Can you work these out from the model? Positions are in its coordinate system, mm. Give positions to 0.01 mm unless a question says otherwise; leave off trailing zeros. Order: outer loops, then holes, each group sorted by start corner. A loop starts at its lowest first (then second) coordinate and runs counter-clockwise, first axis right, second up. Notation, with made-up numbers: (63.25, 75.25) - (83.25, 75.25) arc R15 cw to (83.25, 104.25) - close; hole circle Ø4 at (39.5, 79.25). An arc over 180 degrees is marked (long way). Use one line per item in the form item = value. Start each with the question number.
1) Suppose I cut it at C-C, the plane y = 1405. Write out the boundary of the cut face in (x, z), and give its area (3 significant figures).
2) For pin 1 (10 mm diameter, centred on y = 260, z = 84, fed in from -X); pin 2 (2 mm diameter, centred on x = 2.5, y = 1288, fed in from +Z); pin 3 (1 mm diameter, centred on y = 208.5, z = -30, fed in from -X), each with a flat end and sliding along its axis, tell me the tip position at first contact or that it passes through.
3) Please list where these lines run through material, in increasing order: probe 1 along X at (y, z) = (1181, -28.5); probe 2 along X at (y, z) = (198, -17.5); probe 3 along Z at (x, y) = (-104, 310).
4) Suppose I cut it at B-B, the plane x = 101. Write out the boundary of the cut face in (y, z), and give its area (3 significant figures).
5) Suppose I cut it at D-D, the plane x = 0. Write out the boundary of the cut face in (y, z).
6) Suppose I cut it at A-A, the plane z = -27. Write out the boundary of the cut face in (x, y).
```python
from build123d import *

# Parameters (mm, degrees)
BOSS_EXTRUDE1_DEPTH = 1510


with BuildPart() as part:
    # Sketch2 → Boss-Extrude1 (new body)
    with BuildSketch(Plane(origin=(0, 0, 0), x_dir=(1, 0, 0), z_dir=(0, 1, 0))):
        with BuildLine():
            ThreePointArc((70.554092404, 97.067605539), (106.926355704, 54.467921346), (120, 0))
            Line((120, 0), (125, 0))
            ThreePointArc((125, 0), (111.381620526, 56.737418069), (73.493846254, 101.112089103))
            Line((73.493846254, 101.112089103), (70.554092404, 97.067605539))
        make_face()
        with BuildLine():
            Line((-125, 0), (-120, 0))
            ThreePointArc((-120, 0), (-114.122987747, 37.093714665), (-97.067605539, 70.554092404))
            Line((-97.067605539, 70.554092404), (-101.112089103, 73.493846254))
            ThreePointArc((-101.112089103, 73.493846254), (-118.878112237, 38.63928611), (-125, 0))
        make_face()
        with BuildLine():
            Line((125, 0), (120, 0))
            ThreePointArc((120, 0), (0, -120), (-120, 0))
            Line((-120, 0), (-125, 0))
            ThreePointArc((-125, 0), (0, -125), (125, 0))
        make_face()
    extrude(amount=BOSS_EXTRUDE1_DEPTH)


solid = part.part
```
Result sheet:
q1.outline = (-101.11, -73.49) - (-97.07, -70.55) arc R120 cw (long way) to (70.55, -97.07) - (73.49, -101.11) arc R125 ccw (long way) to start
q1.area = 2,890 mm²
q2.pin_1 = -96.87
q2.pin_2 = 124.99
q2.pin_3 = -121.47
q3.probe_1 = -121.71 to -116.57, 116.57 to 121.71
q3.probe_2 = -123.77 to -118.72, 118.72 to 123.77
q3.probe_3 = -69.35 to -59.87, 59.87 to 69.35
q4.outline = (0, -73.65) - (1510, -73.65) - (1510, -64.8) - (0, -64.8) - close; (0, 64.8) - (1510, 64.8) - (1510, 73.65) - (0, 73.65) - close
q4.area = 26,700 mm²
q5.outline = (0, 120) - (1510, 120) - (1510, 125) - (0, 125) - close
q6.outline = (-122.05, 0) - (-116.92, 0) - (-116.92, 1510) - (-122.05, 1510) - close; (116.92, 0) - (122.05, 0) - (122.05, 1510) - (116.92, 1510) - close
